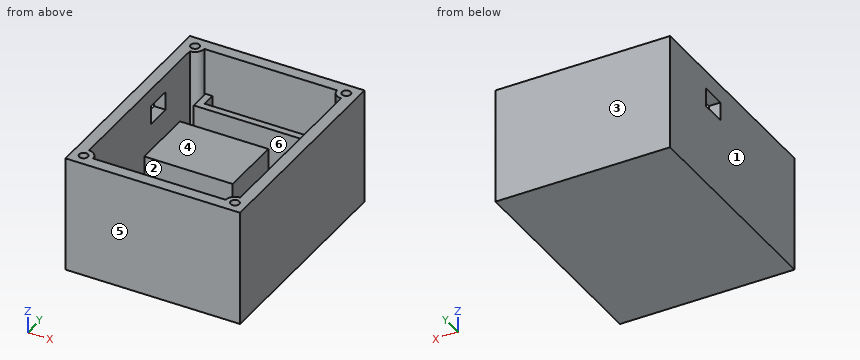
from build123d import *

# Parameters (mm, degrees)
SKETCH1_W           = 95.25
SKETCH1_H           = 120.65
BOSS_EXTRUDE1_DEPTH = 63.5
SHELL1_T            = -6.35
BOSS_EXTRUDE2_DEPTH = 57.15
SKETCH5_R           = 1.905
SKETCH5_W           = 22.2885
SKETCH5_H           = 5.08
BOSS_EXTRUDE5_DEPTH = 6.35
SKETCH7_R           = 1.016
BOSS_EXTRUDE6_DEPTH = 8.89
SKETCH8_R           = 2.38125
CUT_EXTRUDE1_DEPTH  = 8.89
BOSS_EXTRUDE7_DEPTH = 6.35
CUT_EXTRUDE3_REACH  = 97.25
SKETCH13_W          = 10.16
SKETCH13_H          = 13.97
BOSS_EXTRUDE8_DEPTH = 31.75
SKETCH16_W          = 48.26
SKETCH16_H          = 34.544
BOSS_EXTRUDE9_DEPTH = 25.4


with BuildPart() as part:
    # Sketch1 → Boss-Extrude1 (new body)
    with BuildSketch(Plane.XY):
        Rectangle(SKETCH1_W, SKETCH1_H)
    extrude(amount=BOSS_EXTRUDE1_DEPTH)

    # Shell1
    shell1_openings = [part.faces().sort_by_distance(p)[0] for p in [
        (0, 0, 63.5),
    ]]
    offset(amount=SHELL1_T, openings=shell1_openings, kind=Kind.INTERSECTION)

    # Sketch2 → Boss-Extrude2 (add)
    with BuildSketch(Plane.XY.offset(63.5)):
        with BuildLine():
            Line((-41.275, 53.975), (-36.195, 53.975))
            ThreePointArc((-36.195, 53.975), (-37.682897552, 50.382897552), (-41.275, 48.895))
            Line((-41.275, 48.895), (-41.275, 53.975))
        make_face()
        with BuildLine():
            Line((36.195, 53.975), (41.275, 53.975))
            Line((41.275, 53.975), (41.275, 48.895))
            ThreePointArc((41.275, 48.895), (37.682897552, 50.382897552), (36.195, 53.975))
        make_face()
        with BuildLine():
            Line((41.275, -48.895), (41.275, -53.975))
            Line((41.275, -53.975), (36.195, -53.975))
            ThreePointArc((36.195, -53.975), (37.682897552, -50.382897552), (41.275, -48.895))
        make_face()
        with BuildLine():
            Line((-41.275, -48.895), (-41.275, -53.975))
            Line((-41.275, -53.975), (-36.195, -53.975))
            ThreePointArc((-36.195, -53.975), (-37.682897552, -50.382897552), (-41.275, -48.895))
        make_face()
    extrude(amount=-BOSS_EXTRUDE2_DEPTH)

    # Sketch5 → Boss-Extrude5 (add)
    with BuildSketch(Plane.XY.offset(6.35)):
        with Locations((13.2715, -45.085)):
            Circle(SKETCH5_R)
        with Locations((31.75, -45.085)):
            Circle(SKETCH5_R)
        with Locations((22.51075, -23.495)):
            Rectangle(SKETCH5_W, SKETCH5_H)
    extrude(amount=BOSS_EXTRUDE5_DEPTH)

    # Sketch7 → Boss-Extrude6 (add)
    with BuildSketch(Plane.XY.offset(12.7)):
        with Locations((13.2715, -45.085)):
            Circle(SKETCH7_R)
        with Locations((31.75, -45.085)):
            Circle(SKETCH7_R)
    extrude(amount=BOSS_EXTRUDE6_DEPTH)

    # Sketch8 → Cut-Extrude1 (cut)
    with BuildSketch(Plane.XY.offset(63.5)):
        with Locations((-41.275, 53.975)):
            Circle(SKETCH8_R)
        with Locations((41.275, 53.975)):
            Circle(SKETCH8_R)
        with Locations((41.275, -53.975)):
            Circle(SKETCH8_R)
        with Locations((-41.275, -53.975)):
            Circle(SKETCH8_R)
    extrude(amount=-CUT_EXTRUDE1_DEPTH, mode=Mode.SUBTRACT)

    # Sketch10 → Boss-Extrude7 (add)
    with BuildSketch(Plane.XY.offset(6.35)):
        Polygon((-30.8991, -43.307), (-30.8991, -9.7028), (5.0165, -9.7028), (5.0165, -43.307), (-0.0635, -43.307), (-0.0635, -14.7828), (-25.8191, -14.7828), (-25.8191, -43.307), align=None)
    extrude(amount=BOSS_EXTRUDE7_DEPTH)

    # Sketch13 → Cut-Extrude3 (cut, up to next)
    with BuildSketch(Plane.ZY.offset(47.625), mode=Mode.PRIVATE) as cut_extrude3_sk1:
        with Locations((48.768, 18.415)):
            Rectangle(SKETCH13_W, SKETCH13_H)
    cut_extrude3_tool1 = extrude(cut_extrude3_sk1.sketch, amount=-CUT_EXTRUDE3_REACH, mode=Mode.PRIVATE) & part.part
    add(cut_extrude3_tool1.solids().sort_by_distance((-47.625, 18.415, 48.768))[0], mode=Mode.SUBTRACT)

    # Sketch15 → Boss-Extrude8 (add)
    with BuildSketch(Plane.XY.offset(6.35)):
        Polygon((-31.75, 53.975), (-31.75, 46.355), (31.75, 46.355), (31.75, 53.975), (35.56, 53.975), (35.56, 42.545), (-35.56, 42.545), (-35.56, 53.975), align=None)
    extrude(amount=BOSS_EXTRUDE8_DEPTH)

    # Sketch16 → Boss-Extrude9 (add)
    with BuildSketch(Plane.XY.offset(6.35)):
        with Locations((-15.113, 18.415)):
            Rectangle(SKETCH16_W, SKETCH16_H)
    extrude(amount=BOSS_EXTRUDE9_DEPTH)


solid = part.part
Can you work these out from the model? Positions are in its coordinate system, mm. Face numbers are marked on the shaded views. A direction names the side the tool comes from. Give positions to 0.01 mm unless a question says otherwise; leave off trailing zeros. Order: outer loops, then holes, each group sorted by start corner. A loop starts at its lowest first (then second) coordinate and runs counter-clockwise, first axis right, second up. Notation, with made-up numbers: M 31,-28 L 37,-28 A19 ccw 37,-17 Z; hole C -23,77 d5. An arc over 180 degrees is marked long. Use a Markdown table: item, result. Add a question column.
Item 1: Will these pins go through, and if not, where does the flat tip stop? pin 1 (1.4 mm diameter, centred on x = -42, y = -54, fed in from +Z); pin 2 (17.5 mm diameter, centred on x = -12.5, y = 25.5, fed in from +Z); pin 3 (8 mm diameter, centred on x = -19, y = -38, fed in from +Z).
Item 2: Suppose I cut it at C-C (z = 52.5). List the corners of the cut face in (x, y) for me (3 decimals), then the cut area to 3 significant figures.
Item 3: If I drill on L1, parallel to Y at x = -7, z = 35 (3 decimals); L2, parallel to Y at x = -22, z = 10 (3 decimals); L3, parallel to X at y = 44, z = 22 (3 decimals), over which ranges is the centre line in solid material (lowest first)? Write a range as [from, to].
Item 4: Suppose I cut it at B-B (x = -19). List the corners of the cut face in (y, z) for me (3 decimals), then the cut area to 3 significant figures.
Item 5: For the marked faces 5 and 6, which set-ups out of +Z, -Z, +X, -X, +Y, -Y let a thin tool reach every point of the face, with its end or its side?
Item 6: We'd pull the mould along X, two halves only. Please class the marked faces 1, 2, 3 and 4: +X half, -X half, draft (parallel to the pull), parting line (faces both ways), or undercut.
Item 7: Suppose I cut it at A-A (z = 30). List the corners of the cut face in (x, y) for me (3 decimals).
Answer sheet:
| question | item | result |
|---|---|---|
| 1 | pin 1 | stops at z = 54.61 |
| 1 | pin 2 | stops at z = 31.75 |
| 1 | pin 3 | stops at z = 6.35 |
| 2 | outline | M -47.625,-60.325 L 47.625,-60.325 L 47.625,60.325 L -47.625,60.325 L -47.625,25.4 L -41.275,25.4 L -41.275,48.895 A5.08 ccw -36.195,53.975 L 36.195,53.975 A5.08 ccw 41.275,48.895 L 41.275,-48.895 A5.08 ccw 36.195,-53.975 L -36.195,-53.975 A5.08 ccw -41.275,-48.895 L -41.275,11.43 L -47.625,11.43 Z |
| 2 | area | 2,570 mm² |
| 3 | L1 | y = [-60.325, -53.975], [42.545, 46.355], [53.975, 60.325] |
| 3 | L2 | y = [-60.325, -53.975], [-14.783, -9.703], [1.143, 35.687], [42.545, 46.355], [53.975, 60.325] |
| 3 | L3 | x = [-47.625, -41.275], [-35.56, 35.56], [41.275, 47.625] |
| 4 | outline | M -60.325,0 L 60.325,0 L 60.325,63.5 L 53.975,63.5 L 53.975,6.35 L 46.355,6.35 L 46.355,38.1 L 42.545,38.1 L 42.545,6.35 L 35.687,6.35 L 35.687,31.75 L 1.143,31.75 L 1.143,6.35 L -9.703,6.35 L -9.703,12.7 L -14.783,12.7 L -14.783,6.35 L -53.975,6.35 L -53.975,63.5 L -60.325,63.5 Z |
| 4 | area | 2,520 mm² |
| 5 | face 5 | +Z, -Z, +X, -X, -Y |
| 5 | face 6 | +Z |
| 6 | face 1 | -X half |
| 6 | face 2 | undercut |
| 6 | face 3 | draft |
| 6 | face 4 | undercut |
| 7 | outline | M -47.625,-60.325 L 47.625,-60.325 L 47.625,60.325 L -47.625,60.325 Z; M -39.243,1.143 L 9.017,1.143 L 9.017,35.687 L -39.243,35.687 Z; hole M -41.275,-48.895 A5.08 cw -36.195,-53.975 L 36.195,-53.975 A5.08 cw 41.275,-48.895 L 41.275,48.895 A5.08 cw 36.195,53.975 L 35.56,53.975 L 35.56,42.545 L -35.56,42.545 L -35.56,53.975 L -36.195,53.975 A5.08 cw -41.275,48.895 Z; hole M -31.75,46.355 L 31.75,46.355 L 31.75,53.975 L -31.75,53.975 Z |
